```python
from build123d import *

# Parameters (mm, degrees)
ESTRUSIONE_ESTRUSIONE1_DEPTH = 32
SCHIZZO2_R                   = 1
ESTRUSIONE_ESTRUSIONE2_DEPTH = 5
ESTRUSIONE_ESTRUSIONE3_START = 3
SCHIZZO4_R                   = 1
ESTRUSIONE_ESTRUSIONE3_DEPTH = 3


with BuildPart() as part:
    # Schizzo1 → Estrusione-Estrusione1 (new body)
    with BuildSketch(Plane.XY):
        Polygon((0, -16.964772049), (-2.5, -18.408147722), (-2.5, -21.294899068), (0, -22.738274741), (2.5, -21.294899068), (2.5, -18.408147722), align=None)
    extrude(amount=ESTRUSIONE_ESTRUSIONE1_DEPTH)

    # Schizzo2 → Estrusione-Estrusione2 (add)
    with BuildSketch(Plane.XY.offset(32)):
        with Locations((0, -19.851523395)):
            Circle(SCHIZZO2_R)
    extrude(amount=ESTRUSIONE_ESTRUSIONE2_DEPTH)

    # Schizzo4 → Estrusione-Estrusione3 (add)
    with BuildSketch(Plane(origin=(0, 0, 0), x_dir=(-1, 0, 0), z_dir=(0, 0, -1)).offset(ESTRUSIONE_ESTRUSIONE3_START)):
        with Locations(Location((0, -19.851523395, 0), (0, 0, 180))):
            Circle(SCHIZZO4_R)
    extrude(amount=-ESTRUSIONE_ESTRUSIONE3_DEPTH)


solid = part.part
```
Geometry check sheet. Reference: the model listing, model coordinates, mm. A direction names the side the tool comes from. Coordinates: 2 decimals unless noted, no trailing zeros. Order: outer loops, then holes, each group sorted by start corner. A loop starts at its lowest first (then second) coordinate and runs counter-clockwise, first axis right, second up.
Q1. Sectioned sample at C-C on x = 2. Record the cut outline in (y, z).
Reply:
outline: (-21.58, 0) - (-18.12, 0) - (-18.12, 32) - (-21.58, 32) - close
Q2. Thickness scan on probe 1 along Z at (x, y) = (2.25, -20.95); probe 2 along X at (y, z) = (-18.2, 10); probe 3 along Y at (x, z) = (1.9, 31). Record the ranges inside material, lowest first.
Reply:
probe 1: z = 0 to 32
probe 2: x = -2.14 to 2.14
probe 3: y = -21.64 to -18.06
Q3. Depth check by flat-ended pin: pin 1 Ø2 at (y, z) = (-22, 7) entering from +X. Enter the tip coordinate at first touch or a pass-through.
Reply:
pin 1: stops at x = 2.5
Q4. Tool access check on faces 1 (the face through (0.46, -20.74, 34.47)), 2 (the face through (-1.233, -17.676, 15.776)), 3 (the face through (0, -21.1, 0)). Record the directions out of +Z, -Z, +X, -X, +Y, -Y that give a thin tool (end or side, any length) a straight path to the whole face; none if there is none.
Reply:
face 1: +Z
face 2: +Z, -Z, -X, +Y
face 3: -Z
Q5. Sectioned sample at A-A on z = 29. Record the cut outline in (x, y), and give its area (3 significant figures).
Reply:
outline: (-2.5, -21.29) - (0, -22.74) - (2.5, -21.29) - (2.5, -18.41) - (0, -16.96) - (-2.5, -18.41) - close
area: 21.7 mm2
Q6. Sectioned sample at B-B on y = -18. Record the cut outline in (x, z), and give its area (3 significant figures).
Reply:
outline: (-1.79, 0) - (1.79, 0) - (1.79, 32) - (-1.79, 32) - close
area: 115 mm2
